Geometry: final body of the model. Coordinates: model frame, mm. A direction names the side the tool comes from. Give positions to 0.01 mm unless a question says otherwise; leave off trailing zeros. Order: outer loops, then holes, each group sorted by start corner. A loop starts at its lowest first (then second) coordinate and runs counter-clockwise, first axis right, second up. Notation, with made-up numbers: (-14, 81.5) - (39, 81.5) arc R24 cw to (39, 116.5) - close; hole circle Ø7 at (62, 6). An arc over 180 degrees is marked (long way). Write item = value, one per line. Start each with the question number.
from build123d import *

# Parameters (mm, degrees)
SKETCH1_W           = 15
SKETCH1_H           = 30
BOSS_EXTRUDE1_DEPTH = 100
SKETCH2_R           = 10
BOSS_EXTRUDE2_DEPTH = 180
FILLET1_R           = 2


with BuildPart() as part:
    # Sketch1 → Boss-Extrude1 (new body)
    with BuildSketch(Plane(origin=(0, 0, 0), x_dir=(0, 0, -1), z_dir=(1, 0, 0))):
        with Locations((7.5, 15)):
            Rectangle(SKETCH1_W, SKETCH1_H)
    extrude(amount=-BOSS_EXTRUDE1_DEPTH)

    # Sketch2 → Boss-Extrude2 (add)
    with BuildSketch(Plane(origin=(0, 0, -15), x_dir=(-1, 0, 0), z_dir=(0, 0, -1))):
        with Locations((85, 15)):
            Circle(SKETCH2_R)
    extrude(amount=BOSS_EXTRUDE2_DEPTH)

    # Fillet1
    fillet1_edges = [part.edges().sort_by_distance(p)[0] for p in [
        (-75, 15, -15),
    ]]
    fillet(fillet1_edges, radius=FILLET1_R)


solid = part.part
Q1. Section A-A, the plane y = 15. Return the cut outline in (x, z).
Q2. Section B-B, the plane x = -85. Return the cut outline in (y, z), then the cut area to 3 significant figures.
Q3. Contact query for flat-ended pins moving along their axis: pin 1 (2 mm diameter, centred on y = 20.5, z = -94.5, fed in from +X); pin 2 (12 mm diameter, centred on x = -23, y = 14, fed in from -Z); pin 3 (6 mm diameter, centred on y = 13.5, z = -31.5, fed in from +X). Output: stop coordinate, or through.
Q4. Set-up query: faces 1 (the flat face through (-49, 15, 0)), 2 (the cylindrical face through (-75, 15, -105)). Return all of +Z, -Z, +X, -X, +Y, -Y with unobstructed straight access to the full face (end or side cutting, diameter ignored); none if empty.
Q5. Material intervals for line 1 along Z through (x, y) = (-75.5, 1.75); line 2 along X through (y, z) = (21.75, -54.5); line 3 along X through (y, z) = (12.5, -143), sorted ascending. Write a range as from..to.
Q6. Section D-D, the plane x = -7. Return the cut outline in (y, z), then the cut area to 3 significant figures.
Q7. Section C-C, the plane z = -155. Return the cut outline in (x, y), then the cut area to 3 significant figures.
The answers:
q1.outline = (-100, -15) - (-97, -15) arc R2 cw to (-95, -17) - (-95, -195) - (-75, -195) - (-75, -17) arc R2 cw to (-73, -15) - (0, -15) - (0, 0) - (-100, 0) - close
q2.outline = (0, -15) - (3, -15) arc R2 cw to (5, -17) - (5, -195) - (25, -195) - (25, -17) arc R2 cw to (27, -15) - (30, -15) - (30, 0) - (0, 0) - close
q2.area = 4,050 mm²
q3.pin_1 = -76.07
q3.pin_2 = -15
q3.pin_3 = -75
q4.face_1 = +Z, +X, -X, +Y, -Y
q4.face_2 = -Z
q5.line_1 = -15..0
q5.line_2 = -92.38..-77.62
q5.line_3 = -94.68..-75.32
q6.outline = (0, -15) - (30, -15) - (30, 0) - (0, 0) - close
q6.area = 450 mm²
q7.outline = circle Ø20 at (-85, 15)
q7.area = 314 mm²
